```python
from build123d import *

# Parameters (mm, degrees)
F0_R     = 26.67
F1_DEPTH = 101.6
F2_SIZE2 = 52.3394448406
F2_SIZE  = 19.05
F3_R     = 5.0165
F4_DEPTH = 101.6
F5_DEPTH = 25.4


with BuildPart() as f1:
    # F0 (on Top) → F1 (new body)
    with BuildSketch(Plane.XY):
        Circle(F0_R)
    extrude(amount=F1_DEPTH)

    # F2
    f2_edges = [f1.edges().sort_by_distance(p)[0] for p in [
        (-26.67, 0, 101.6),
    ]]
    f2_side = f1.faces().sort_by_distance((0, 0, 101.6))[0]
    chamfer(f2_edges, length=F2_SIZE, length2=F2_SIZE2, reference=f2_side)

    # F3 (on face) → F4 (cut)
    with BuildSketch(Plane(origin=(0, 0, 0), x_dir=(1, 0, 0), z_dir=(0, 0, -1))):
        Circle(F3_R)
    extrude(amount=-F4_DEPTH, mode=Mode.SUBTRACT)

    # F5 (add): a face of the model
    f5_faces = [f1.faces().sort_by_distance(p)[0] for p in [
        (-25.9156584858, 0, 0),
    ]]
    extrude(f5_faces, amount=F5_DEPTH)


solid = f1.part
```
Read the model definition and answer for the solid it produces. Units are mm, in the model's axes. Give positions to 0.01 mm unless a question says otherwise; leave off trailing zeros. Order: outer loops, then holes, each group sorted by start corner. A loop starts at its lowest first (then second) coordinate and runs counter-clockwise, first axis right, second up.
(1) Given pin 1 (1 mm diameter, centred on x = 0.5, z = 9, fed in from -Y); pin 2 (1.5 mm diameter, centred on x = 5.5, z = 31.5, fed in from +Y); pin 3 (5 mm diameter, centred on x = 4.5, y = 6.5, fed in from +Z); pin 4 (10 mm diameter, centred on x = -5.5, z = 69.5, fed in from -Y), each flat-ended and moving along its own axis, determine where each tip first touches the part or whether it passes through.
(2) Find section A-A (y = 0). Give the vertices of the cut face in (x, z).
(3) Straight lines are drawn through the part: L1, parallel to Y at x = 0, z = 29; L2, parallel to X at y = 4.5, z = 71.5; L3, parallel to X at y = 0, z = 56. For each, find the intervals that lie inside material, in ascending order.
(4) For a pull along X with two mould halves and no side action, classify faces 1 (the cylindrical face through (-3.472, 26.443, 12.453)), 2 (the flat face through (2, -5, 101.6)), 3 (the cylindrical face through (-1.087, 4.897, 38.989)) as released by +X, released by -X, zero draft, split by the parting line, or undercut.
(5) Find section C-C (z = 43.5). Give the vertices of the cut face in (x, y).
(6) Find section D-D (z = 84.5). Give the vertices of the cut face in (x, y).
Result sheet:
1. pin 1: stops at y = -26.67
1. pin 2: stops at y = 26.24
1. pin 3: stops at z = 101.6
1. pin 4: stops at y = -20.68
2. outline: (-26.67, -25.4) - (-5.02, -25.4) - (-5.02, 101.6) - (-7.62, 101.6) - (-26.67, 49.26) - close; (5.02, -25.4) - (26.67, -25.4) - (26.67, 49.26) - (7.62, 101.6) - (5.02, 101.6) - close
3. L1: y = -26.67 to -5.02, 5.02 to 26.67
3. L2: x = -18.02 to -2.22, 2.22 to 18.02
3. L3: x = -24.22 to -5.02, 5.02 to 24.22
4. face 1: split by the parting line
4. face 2: zero draft
4. face 3: undercut
5. outline: circle Ø53.34 at (0, 0); hole circle Ø10.03 at (0, 0)
6. outline: circle Ø27.69 at (0, 0); hole circle Ø10.03 at (0, 0)
